Autodesk Fusion 360 part; units mm, degrees
sketch "Sketch2" plane through (0, 0, 0) normal (0, 0, 1) x (1, 0, 0)
  circle A0 centre (0, 0) radius 46
  circle A1 centre (0, 0) radius 25
  line L0 (0, 1.75) -> (0, 22.5) construction
  circle A2 centre (0, 0) radius 36
  point P0 (-41, 0)
  point P1 (41, 0)
  dimension "d4" = 50
  dimension "d5" = 82
  dimension "d6" = 92
  dimension "d7" = -10
extrude "Extrude1" add sketch "Sketch2" against normal blind 35 contours A0
extrude "Extrude2" add sketch "Sketch2" against normal blind 10 contours A2
hole "Hole1" at (-41, 0, 0) at (41, 0, 0) direction (0, 0, -1) diameter 5.035 depth 10 tip angle 118
sketch "Sketch3" plane through (0, 0, 0) normal (1, 0, 0) x (0, 0, -1)
  line L0 (10, 46) -> (10, 39)
  line L1 (10, 39) -> (25, 39)
  line L2 (25, 39) -> (25, 40)
  line L3 (25, 40) -> (35, 40)
  line L4 (-1.75, 0) -> (-22.5, 0) construction
  line L5 (35, -46) -> (35, 46)
  line L6 (0, 46) -> (0, -46)
  line L7 (35, 46) -> (10, 46)
  dimension "d15" = 40
  dimension "d16" = 1
  dimension "d17" = 25
  dimension "d18" = 10
revolve "Revolve1" cut sketch "Sketch3" angle 360 about axis through (0, 0, 1.75) along (0, 0, 1)
chamfer "Chamfer1" distance 1 angle 45 4 edges at (-42.8871, -16.6343, 0) (-42.8871, -16.6343, -10) (-14.4646, -37.2931, -35) (-23.3082, 9.0404, 0)
For this review, take the finished solid that the model builds, in its own axes (mm). A direction names the side the tool comes from. Round coordinates to 2 decimals unless told otherwise and drop trailing zeros. Order: outer loops, then holes, each group sorted by start corner. A loop starts at its lowest first (then second) coordinate and runs counter-clockwise, first axis right, second up.
Q1. We need section C-C, the plane y = 0. State how many separate pieces and enclosed holes the cut face has, plus the area to 3 significant figures.
Findings below:
separate pieces: 4
enclosed holes: 0
area: 485 mm2
Q2. We need section D-D, the plane z = -22.5. Give the boundary of the cut face in (x, y), plus the area to 3 significant figures.
Findings below:
outline: circle Ø78 at (0, 0); hole circle Ø72 at (0, 0)
area: 707 mm2
Q3. Mouldability with a two-part tool opening along X and no side actions: class faces 6 (the cylindrical face through (-5.99, 45.61, -4.94)), 7 (the flat face through (11.4, -34.5, -35)), 8 (the cylindrical face through (-4.686, 35.694, -22.325)) as pulls with the +X half, pulls with the -X half, needs draft (parallel to the pull), parting line crosses it, or undercut.
Findings below:
face 6: parting line crosses it
face 7: needs draft
face 8: undercut
Q4. Machinability: for faces 1 (the flat face through (-25, -7, -10)), 2 (the flat face through (19, -19, 0)), 3 (the cylindrical face through (38.668, -5.077, -17.605)), 4 (the cylindrical face through (38.5, 0.3, -5.1)), 5 (the cylindrical face through (23.846, 7.509, -5.437)), which of the approach directions +Z, -Z, +X, -X, +Y, -Y give a long, thin tool a straight path to every point of the face, cutting with its end or side? Answer none if there is none.
Findings below:
face 1: -Z
face 2: +Z, +X, -X, +Y, -Y
face 3: none
face 4: +Z
face 5: +Z, -Z
Q5. Wall thickness on line 1 (Y direction, x = 0, z = -5.5); line 2 (Z direction, x = -11, y = -33.5); line 3 (Y direction, x = 15.5, z = -23.5): over which ranges is each line inside the solid? List them lowest first.
Findings below:
line 1: y = -46 to -25, 25 to 46
line 2: z = -10 to 0
line 3: y = -35.79 to -32.49, 32.49 to 35.79
Q6. We need section B-B, the plane z = -7.5. Give the boundary of the cut face in (x, y) (1 decimal), plus the area to 3 significant figures.
Findings below:
outline: circle Ø92 at (0, 0); hole circle Ø5 at (-41, 0); hole circle Ø50 at (0, 0); hole circle Ø5 at (41, 0)
area: 4,640 mm2
Q7. Insertion check: P1, Ø8, axis at x = 41, y = 0, coming from the +Z side; P2, Ø6, axis at y = 7.5, z = -23, coming from the +X side; P3, Ø10, axis at x = -27, z = -27, coming from the +Y side; P4, Ø3, axis at x = 10, y = -28.5, coming from the -Z side. Each pin has a flat end and moves straight along its axis. Give the tip position at first contact, or say it passes through.
Findings below:
P1: stops at z = 0
P2: stops at x = 39.65
P3: stops at y = 33.41
P4: stops at z = -10
Q8. We need section A-A, the plane x = 0. Give the boundary of the cut face in (y, z).
Findings below:
outline: (-46, -9) - (-45, -10) - (-39, -10) - (-39, -25) - (-40, -25) - (-40, -34) - (-39, -35) - (-36, -35) - (-36, -10) - (-25, -10) - (-25, -1) - (-26, 0) - (-45, 0) - (-46, -1) - close; (25, -10) - (36, -10) - (36, -35) - (39, -35) - (40, -34) - (40, -25) - (39, -25) - (39, -10) - (45, -10) - (46, -9) - (46, -1) - (45, 0) - (26, 0) - (25, -1) - close
